Geometry: final body of the model. Coordinates: model frame, mm. Face numbers are marked on the shaded views. A direction names the side the tool comes from. Round coordinates to 2 decimals unless told otherwise and drop trailing zeros. Loops run counter-clockwise (first coordinate to the right, second up) from the corner with the lowest first, then second, coordinate; pieces in that order, holes last. Notation, with made-up numbers: (60.25, 5.25) -> (69.25, 5.25) arc R11 cw to (69.25, 22.25) -> close; hole circle Ø7 at (69.5, 17). An arc over 180 degrees is marked (long way). Answer in a Markdown table with one row per item.
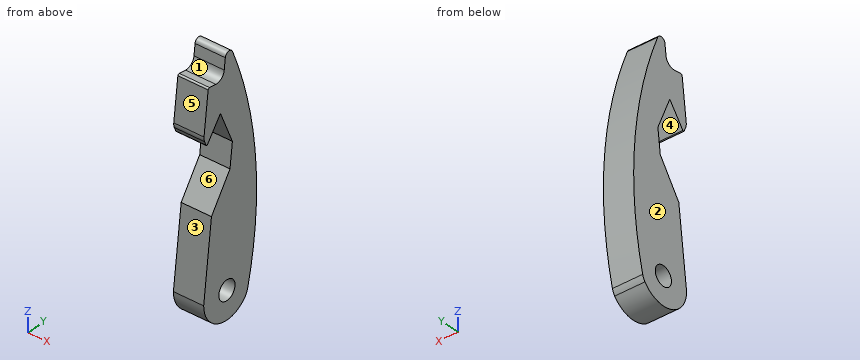
```python
from build123d import *

# Parameters (mm, degrees)
SKETCH2_R           = 1.6
BOSS_EXTRUDE1_DEPTH = 5
FILLET2_R           = 1.5
CHAMFER1_SIZE       = 2.5
CHAMFER1_SIZE2      = 1.443375673
FILLET3_R           = 1.5
FILLET4_R           = 0.25
FILLET5_R           = 0.15
FILLET6_R           = 0.75
FILLET7_R           = 2.5


with BuildPart() as part:
    # Sketch2 → Boss-Extrude1 (new body)
    with BuildSketch(Plane.YZ):
        with BuildLine():
            Line((0, 38.5), (-0.711820293, 32.542373638))
            Line((-0.711820293, 32.542373638), (-3.690633474, 32.898283784))
            Line((-3.690633474, 32.898283784), (-4.877000628, 22.968906514))
            Line((-4.877000628, 22.968906514), (-1.281732991, 27.772452143))
            Line((-1.281732991, 27.772452143), (1.080625734, 22.257086221))
            Line((1.080625734, 22.257086221), (0.606078872, 18.285335313))
            Line((0.606078872, 18.285335313), (-3.061283722, 12.878386238))
            Line((-3.061283722, 12.878386238), (-4.6, 0))
            ThreePointArc((-4.6, 0), (-1.190567607, -4.443258801), (3.983716857, -2.3))
            ThreePointArc((3.983716857, -2.3), (5.584415843, 18.450777734), (0, 38.5))
        make_face()
        with Locations(Location((0, 0, 0), (0, 0, 270))):
            Circle(SKETCH2_R, mode=Mode.SUBTRACT)
    extrude(amount=BOSS_EXTRUDE1_DEPTH)

    # Fillet2
    fillet2_edges = [part.edges().sort_by_distance(p)[0] for p in [
        (2.5, -0.711820293, 32.542373638),
    ]]
    fillet(fillet2_edges, radius=FILLET2_R)

    # Chamfer1
    chamfer1_edges = [part.edges().sort_by_distance(p)[0] for p in [
        (2.5, -4.877000628, 22.968906514),
    ]]
    chamfer1_side = [part.faces().sort_by_distance(p)[0] for p in [
        (2.5, -4.283817051, 27.933595149),
    ]]
    chamfer(chamfer1_edges, length=CHAMFER1_SIZE, length2=CHAMFER1_SIZE2, reference=chamfer1_side[0])

    # Fillet3
    fillet3_edges = [part.edges().sort_by_distance(p)[0] for p in [
        (2.5, -4.580408839, 25.451250831),
    ]]
    fillet(fillet3_edges, radius=FILLET3_R)

    # Fillet4
    fillet4_edges = [part.edges().sort_by_distance(p)[0] for p in [
        (2.5, -3.690633474, 32.898283784),
    ]]
    fillet(fillet4_edges, radius=FILLET4_R)

    # Fillet5
    fillet5_edges = [part.edges().sort_by_distance(p)[0] for p in [
        (2.5, -4.012113654, 24.124459998),
    ]]
    fillet(fillet5_edges, radius=FILLET5_R)

    # Fillet6
    fillet6_edges = [part.edges().sort_by_distance(p)[0] for p in [
        (2.5, 0, 38.5),
    ]]
    fillet(fillet6_edges, radius=FILLET6_R)

    # Fillet7
    fillet7_edges = [part.edges().sort_by_distance(p)[0] for p in [
        (2.5, 3.983716857, -2.3),
    ]]
    fillet(fillet7_edges, radius=FILLET7_R)


solid = part.part
```
Item 1: Reachability of the marked faces 4, 5 and 6 from +Z, -Z, +X, -X, +Y, -Y: full face, straight path, thin tool, end or side. Return the list, or none.
Answer:
| item | result |
|---|---|
| face 4 | +X, -X |
| face 5 | +Z, +X, -X, -Y |
| face 6 | +X, -X, -Y |
Item 2: Line query: probe 1 along Z at (x, y) = (1.7, -0.25); probe 2 along Y at (x, z) = (2.1, 0); probe 3 along Z at (x, y) = (3.2, -1.75). Output: solid intervals per line, ascending. Write a range as [from, to].
Answer:
| item | result |
|---|---|
| probe 1 | z = [-4.59, -1.58], [1.58, 17.02], [25.36, 36.06] |
| probe 2 | y = [-4.6, -1.6], [1.6, 4.53] |
| probe 3 | z = [-4.25, 14.81], [27.15, 32.73] |
Item 3: Cut plane B-B (y = 5). Output: boundary loops of the cut face in (x, z).
Answer:
| item | result |
|---|---|
| outline | (0, 2.45) -> (5, 2.45) -> (5, 22.79) -> (0, 22.79) -> close |
Item 4: Pin query (flat end, axial travel): pin 1 Ø3 at (x, y) = (1, -2) entering from -Z; pin 2 Ø1.9 at (y, z) = (0, 0) entering from +X. Return the tip coordinate at first contact, or that it passes through.
Answer:
| item | result |
|---|---|
| pin 1 | stops at z = -4.57 |
| pin 2 | passes through |
Item 5: Draft query along Y for the marked faces 1, 2 and 3. Return one class per face: pulls with the +Y half, pulls with the -Y half, needs draft (parallel to the pull), parting line crosses it, or undercut.
Answer:
| item | result |
|---|---|
| face 1 | undercut |
| face 2 | needs draft |
| face 3 | pulls with the -Y half |
Item 6: Cut plane A-A (z = 10.5). Output: boundary loops of the cut face in (x, y).
Answer:
| item | result |
|---|---|
| outline | (0, -3.35) -> (5, -3.35) -> (5, 5.83) -> (0, 5.83) -> close |
